Design review of the part built by this model. Coordinates are the model's own, in mm. A direction names the side the tool comes from. Coordinates: 2 decimals unless noted, no trailing zeros. Loops run counter-clockwise (first coordinate to the right, second up) from the corner with the lowest first, then second, coordinate; pieces in that order, holes last. Notation, with made-up numbers: M 14.25,56 L 22.25,56 A20 cw 22.25,89 Z; hole C -7,-21.5 d5. An arc over 180 degrees is marked long. Answer as a JSON object with one key per item and string values. Group by question number.
1. Machinability: for faces 1 (the flat face through (-76.2, 0, 2)), 2 (the flat face through (-31.925, 5, 11)), 3 (the flat face through (12.89, 4, 26)), 4 (the cylindrical face through (-33.446, 0.03, 11.632)), 5 (the flat face through (-33, 5, 17.7)), which of the approach directions +Z, -Z, +X, -X, +Y, -Y give a long, thin tool a straight path to every point of the face, cutting with its end or side? Answer none if there is none.
2. To check wall thickness, follow probe 1 along X at (y, z) = (12, 3); probe 2 along Y at (x, z) = (63.5, 2.7); probe 3 along Z at (x, y) = (-5.5, 12). State the ranges of each line that lie inside material, in increasing order.
3. Draft analysis for pull direction Y (two halves, no side actions). For faces 6 (the cylindrical face through (-67.565, 0.179, 2.465)), 7 (the flat face through (6, 19.05, 4)), 8 (the flat face through (-33, -3.175, 11)), state which applies: +Y half, -Y half, draft (parallel to the pull), parting line (faces both ways), or undercut.
4. Consider section C-C (x = 15). State the section outline as (y, z) points, then the cut area to 4 significant figures.
5. Insertion check: pin 1 (3 mm diameter, centred on x = -3.5, y = -5.5, fed in from +Z); pin 2 (10 mm diameter, centred on y = 3, z = 11.5, fed in from +X); pin 3 (3.5 mm diameter, centred on x = -33.5, y = 1, fed in from +Z); pin 4 (5 mm diameter, centred on x = 50.8, y = 9.525, fed in from -Z). Each pin has a flat end and moves straight along its axis. Give the tip position at first contact, or say it passes through.
6. Consider section A-A (x = 50.8). State the section outline as (y, z) points, then the cut area to 3 significant figures.
7. Consider section B-B (x = -63.5). State the section outline as (y, z) points.
from build123d import *

# Parameters (mm, degrees)
F0_W     = 76.2
F0_H     = 38.1
F0_R     = 4.06875
F0_R_2   = 3.175
F1_DEPTH = 5
F2_W     = 4
F2_H     = 19.05
F3_DEPTH = 43.18
F4_W     = 3
F4_H     = 15.875
F5_DEPTH = 12.7
F7_DEPTH = 4
F8_R     = 1.349997
F9_DEPTH = 3


with BuildPart() as f1:
    # F0 (on Top) → F1 (new body)
    with BuildSketch(Plane.XY):
        with Locations((38.1, 0)):
            Rectangle(F0_W, F0_H)
        with Locations((63.5, 0)):
            Circle(F0_R, mode=Mode.SUBTRACT)
        with Locations((50.8, 9.525)):
            Circle(F0_R_2, mode=Mode.SUBTRACT)
        with Locations((-38.1, 0)):
            Rectangle(F0_W, F0_H)
        with Locations((-63.5, 0)):
            Circle(F0_R, mode=Mode.SUBTRACT)
        with Locations((-50.8, 9.525)):
            Circle(F0_R_2, mode=Mode.SUBTRACT)
    extrude(amount=F1_DEPTH)

    # F2 (on face) → F3 (join)
    with BuildSketch(Plane.XY.offset(5)):
        with Locations((10.89, 9.525)):
            Rectangle(F2_W, F2_H)
        with Locations((10.89, -9.525)):
            Rectangle(F2_W, F2_H)
    extrude(amount=F3_DEPTH)

    # F4 (on face) → F5 (join)
    with BuildSketch(Plane.XY.offset(5)):
        with Locations((-33.425, 4.7625)):
            Rectangle(F4_W, F4_H)
    extrude(amount=F5_DEPTH)

    # F6 (on face) → F7 (cut, through all)
    with BuildSketch(Plane.YZ.offset(12.89)):
        with BuildLine():
            Line((-8.099996, 26.59), (1.3e-05, 26.59))
            ThreePointArc((1.3e-05, 26.59), (-8.099996, 34.690009), (-16.200006, 26.59))
            Line((-16.200006, 26.59), (-8.099996, 26.59))
        make_face()
        with BuildLine():
            ThreePointArc((-16.200006, 26.59), (-8.099996, 18.489991), (1.3e-05, 26.59))
            Line((1.3e-05, 26.59), (-8.099996, 26.59))
            Line((-8.099996, 26.59), (-16.200006, 26.59))
        make_face()
        with BuildLine():
            ThreePointArc((0, 46.187605), (-2.199983, 44.08999), (0, 41.992376))
            Line((0, 41.992376), (0, 46.187605))
        make_face()
        with BuildLine():
            Line((0, 46.187605), (0, 41.992376))
            ThreePointArc((0, 41.992376), (1.419874, 42.640851), (2.000009, 44.08999))
            ThreePointArc((2.000009, 44.08999), (1.419874, 45.53913), (0, 46.187605))
        make_face()
        with BuildLine():
            ThreePointArc((2.000009, 9.09001), (1.419874, 10.539149), (0, 11.187624))
            Line((0, 11.187624), (0, 6.992395))
            ThreePointArc((0, 6.992395), (1.419874, 7.64087), (2.000009, 9.09001))
        make_face()
        with BuildLine():
            Line((0, 6.992395), (0, 11.187624))
            ThreePointArc((0, 11.187624), (-2.199983, 9.09001), (0, 6.992395))
        make_face()
    extrude(amount=-F7_DEPTH, mode=Mode.SUBTRACT)

    # F8 (on face) → F9 (cut, through all)
    with BuildSketch(Plane(origin=(-34.925, 0, 0), x_dir=(0, -1, 0), z_dir=(-1, 0, 0))):
        with Locations((-9.787496, 12.949984)):
            Circle(F8_R)
        with Locations((0.262496, 12.949984)):
            Circle(F8_R)
    extrude(amount=-F9_DEPTH, mode=Mode.SUBTRACT)


solid = f1.part
Findings below:
{
 "1": {"face 1": "+Z, -Z, -X, +Y, -Y", "face 2": "+Z, +Y, -Y", "face 3": "+Z, +X, +Y, -Y", "face 4": "-X", "face 5": "+Z, -X, +Y, -Y"},
 "2": {"probe 1": "x = -76.2 to -52.79, -48.81 to 48.81, 52.79 to 76.2", "probe 2": "y = -19.05 to -4.07, 4.07 to 19.05", "probe 3": "z = 0 to 5"},
 "3": {"face 6": "undercut", "face 7": "+Y half", "face 8": "-Y half"},
 "4": {"outline": "M -19.05,0 L 19.05,0 L 19.05,5 L -19.05,5 Z", "area": "190.5 mm^2"},
 "5": {"pin 1": "stops at z = 5", "pin 2": "stops at x = 12.89", "pin 3": "stops at z = 17.7", "pin 4": "passes through"},
 "6": {"outline": "M -19.05,0 L 6.35,0 L 6.35,5 L -19.05,5 Z; M 12.7,0 L 19.05,0 L 19.05,5 L 12.7,5 Z", "area": "159 mm^2"},
 "7": {"outline": "M -19.05,0 L -4.07,0 L -4.07,5 L -19.05,5 Z; M 4.07,0 L 19.05,0 L 19.05,5 L 4.07,5 Z"}
}
